Here's the drawing with two shaded views (mm, measured from the low corner). I have some questions. A direction names the side the tool comes from. Coordinates: 2 decimals unless noted, no trailing zeros. Order: outer loops, then holes, each group sorted by start corner. A loop starts at its lowest first (then second) coordinate and runs counter-clockwise, first axis right, second up. Notation, with made-up numbers: (25.5, 17.25) -> (42.5, 17.25) arc R29 ccw to (42.5, 41.25) -> close; hole circle Ø2 at (54.5, 38.25). An arc over 180 degrees is marked (long way). Write item = value, one per line.
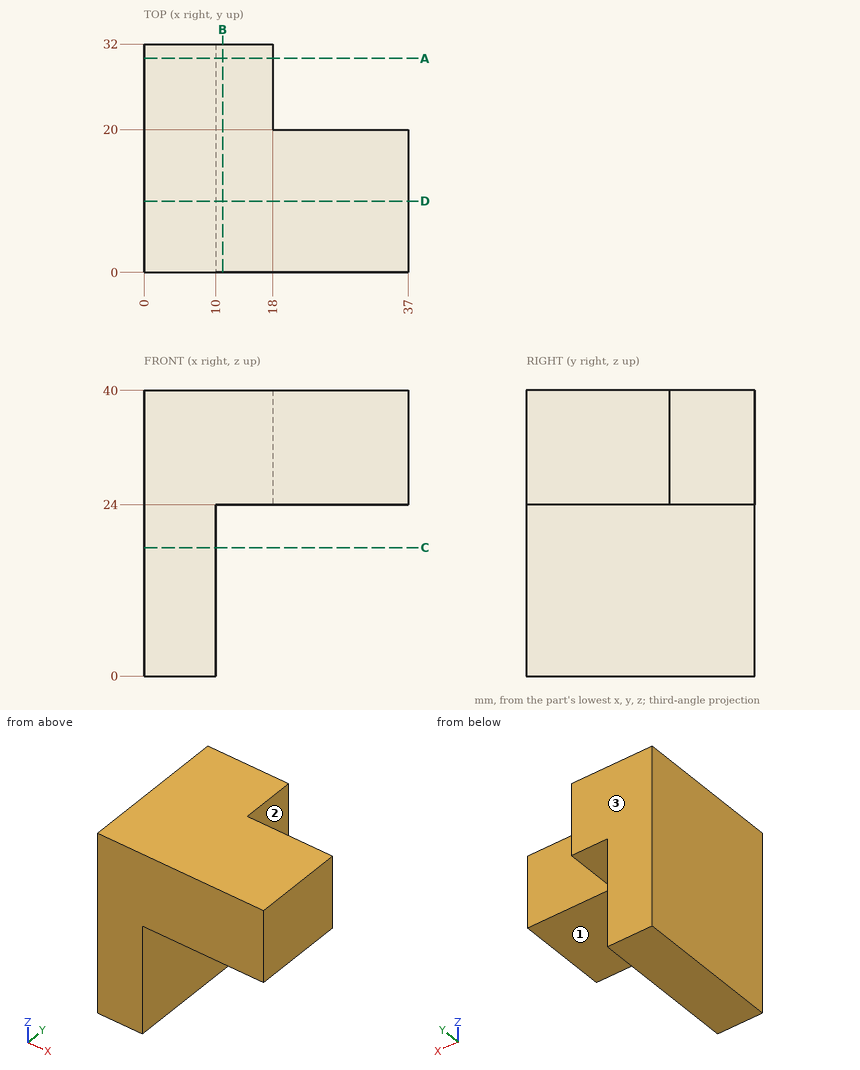
Item 1: I want a section at A-A, the plane y = 30. Please give me the cut outline in (x, z).
A:
outline = (0, 0) -> (10, 0) -> (10, 24) -> (18, 24) -> (18, 40) -> (0, 40) -> close
Item 2: I'm going to push flat-ended pins straight in: P1, Ø12, axis at y = 14, z = 8, coming from the +X side; P2, Ø1.5, axis at y = 7.5, z = 34.5, coming from the -X side; P3, Ø1, axis at x = 12.5, y = 7, coming from the -Z side; P4, Ø1, axis at x = 20.5, z = 33, coming from the +Y side. Where does each tip first touch, or does it pass through?
A:
P1 = 10
P2 = 0
P3 = 24
P4 = 20
Item 3: I want a section at C-C, the plane z = 18. Please give me the cut outline in (x, y).
A:
outline = (0, 0) -> (10, 0) -> (10, 32) -> (0, 32) -> close
Item 4: I want a section at B-B, the plane x = 11. Please give me the cut outline in (y, z).
A:
outline = (0, 24) -> (32, 24) -> (32, 40) -> (0, 40) -> close
Item 5: For the marked faces 1, 2 and 3, which set-ups out of +Z, -Z, +X, -X, +Y, -Y let a thin tool reach every point of the face, with its end or its side?
A:
face_1 = -Z, +X, +Y, -Y
face_2 = +Z, -Z, +X, +Y
face_3 = +Z, -Z, +X, -X, +Y
Item 6: If I drill on probe 1 along Z at (x, y) = (15.5, 21); probe 2 along X at (y, z) = (28.5, 16); probe 3 along Y at (x, z) = (24.5, 31), over which ranges is the centre line in solid material (lowest first)?
A:
probe_1 = 24 to 40
probe_2 = 0 to 10
probe_3 = 0 to 20
Item 7: I want a section at D-D, the plane y = 10. Please give me the cut outline in (x, z), plus the area to 3 significant figures.
A:
outline = (0, 0) -> (10, 0) -> (10, 24) -> (37, 24) -> (37, 40) -> (0, 40) -> close
area = 832 mm2
